from build123d import *

# Parameters (mm, degrees)
SKETCH1_R           = 2.2
BOSS_EXTRUDE1_DEPTH = 5
FILLET1_R           = 3


with BuildPart() as part:
    # Sketch1 → Boss-Extrude1 (new body)
    with BuildSketch(Plane(origin=(0, 0, 0), x_dir=(1, 0, 0), z_dir=(0, 1, 0))):
        with BuildLine():
            Line((0, 10), (43, 10))
            Line((43, 10), (43, 27))
            ThreePointArc((43, 27), (45.343145751, 32.656854249), (51, 35))
            Line((51, 35), (55, 35))
            ThreePointArc((55, 35), (60.656854249, 32.656854249), (63, 27))
            Line((63, 27), (63, 10))
            Line((63, 10), (97, 10))
            Line((97, 10), (97, 27))
            ThreePointArc((97, 27), (99.343145751, 32.656854249), (105, 35))
            Line((105, 35), (109, 35))
            ThreePointArc((109, 35), (114.656854249, 32.656854249), (117, 27))
            Line((117, 27), (117, 10))
            Line((117, 10), (160, 10))
            ThreePointArc((160, 10), (170, 0), (160, -10))
            Line((160, -10), (0, -10))
            ThreePointArc((0, -10), (-10, 0), (0, 10))
        make_face()
        with Locations(Location((53, 27, 0), (0, 0, 270))):
            Circle(SKETCH1_R, mode=Mode.SUBTRACT)
        with Locations(Location((107, 27, 0), (0, 0, 270))):
            Circle(SKETCH1_R, mode=Mode.SUBTRACT)
        with BuildLine():
            Line((5, 2), (155, 2))
            ThreePointArc((155, 2), (157, 0), (155, -2))
            Line((155, -2), (5, -2))
            ThreePointArc((5, -2), (3, 0), (5, 2))
        make_face(mode=Mode.SUBTRACT)
    extrude(amount=BOSS_EXTRUDE1_DEPTH)

    # Fillet1
    fillet1_edges = [part.edges().sort_by_distance(p)[0] for p in [
        (43, 2.5, -10),
        (63, 2.5, -10),
        (97, 2.5, -10),
        (117, 2.5, -10),
    ]]
    fillet(fillet1_edges, radius=FILLET1_R)


solid = part.part
Could you check a few things on this model? Use its own coordinates, in mm. A direction names the side the tool comes from. Give positions to 0.01 mm unless a question says otherwise; leave off trailing zeros. Write each loop counter-clockwise with the first axis right and the second up, starting at its lowest first coordinate (ties: lowest second). Pieces come first, ordered by that corner, then holes. Notation, with made-up numbers: (87, -13.75) -> (129, -13.75) arc R17 cw to (129, 11.25) -> close; hole circle Ø2 at (-23.5, 78.25). An arc over 180 degrees is marked (long way). Answer as a JSON object with one key per item and string values.
Q1. Will these pins go through, and if not, where does the flat tip stop? pin 1 Ø2.5 at (y, z) = (2, -16.5) entering from +X; pin 2 Ø7 at (x, z) = (107, -27) entering from +Y; pin 3 Ø2 at (y, z) = (1.5, -11.5) entering from -X; pin 4 Ø1.5 at (x, y) = (26.5, 2) entering from -Z.
Taken from the geometry:
{"pin 1": "stops at x = 117", "pin 2": "stops at y = 5", "pin 3": "stops at x = 41.66", "pin 4": "stops at z = -10"}
Q2. Suppose I cut it at D-D on x = 141.5. Write out the boundary of the cut face in (y, z).
Taken from the geometry:
{"outline": "(0, -10) -> (5, -10) -> (5, -2) -> (0, -2) -> close; (0, 2) -> (5, 2) -> (5, 10) -> (0, 10) -> close"}
Q3. Which directions (+Z, -Z, +X, -X, +Y, -Y) give clear straight access to the entire face, cutting with the end or side of a thin tool? Please do faces 1 (the flat face through (63, 2, -20)), 2 (the flat face through (20, 2, -10)), 3 (the cylindrical face through (3, 2, 0)).
Taken from the geometry:
{"face 1": "-Z, +Y, -Y", "face 2": "-Z, -X, +Y, -Y", "face 3": "+Y, -Y"}
Q4. Please list where these lines run through material, in increasing order: L1, parallel to X at y = 2.8, z = -27; L2, parallel to Z at x = 73, y = 0.8; L3, parallel to X at y = 0.95, z = -20.
Taken from the geometry:
{"L1": "x = 43 to 50.8, 55.2 to 63, 97 to 104.8, 109.2 to 117", "L2": "z = -10 to -2, 2 to 10", "L3": "x = 43 to 63, 97 to 117"}
Q5. We'd pull the mould along Z, two halves only. Please class faces 4 (the cylindrical face through (50.852, 2.465, -27.477)), 5 (the cylindrical face through (170, 2, 0)), 6 (the flat face through (43, 2, -20)): released by +Z, released by -Z, zero draft, split by the parting line, or undercut.
Taken from the geometry:
{"face 4": "undercut", "face 5": "split by the parting line", "face 6": "zero draft"}
Q6. Suppose I cut it at B-B on x = 107. Write out the boundary of the cut face in (y, z), then the cut area to 3 significant figures.
Taken from the geometry:
{"outline": "(0, -35) -> (5, -35) -> (5, -29.2) -> (0, -29.2) -> close; (0, -24.8) -> (5, -24.8) -> (5, -2) -> (0, -2) -> close; (0, 2) -> (5, 2) -> (5, 10) -> (0, 10) -> close", "area": "183 mm²"}
Q7. Suppose I cut it at C-C on y = 2.35. Write out the boundary of the cut face in (x, z), then the cut area to 3 significant figures.
Taken from the geometry:
{"outline": "(0, -10) -> (40, -10) arc R3 cw to (43, -13) -> (43, -27) arc R8 ccw to (51, -35) -> (55, -35) arc R8 ccw to (63, -27) -> (63, -13) arc R3 cw to (66, -10) -> (94, -10) arc R3 cw to (97, -13) -> (97, -27) arc R8 ccw to (105, -35) -> (109, -35) arc R8 ccw to (117, -27) -> (117, -13) arc R3 cw to (120, -10) -> (160, -10) arc R10 ccw to (160, 10) -> (0, 10) arc R10 ccw to start; hole (5, -2) -> (155, -2) arc R2 ccw to (155, 2) -> (5, 2) arc R2 ccw to start; hole circle Ø4.4 at (53, -27); hole circle Ø4.4 at (107, -27)", "area": "3,820 mm²"}
Q8. Suppose I cut it at A-A on z = 0. Write out the boundary of the cut face in (x, y).
Taken from the geometry:
{"outline": "(-10, 0) -> (3, 0) -> (3, 5) -> (-10, 5) -> close; (157, 0) -> (170, 0) -> (170, 5) -> (157, 5) -> close"}
